Design review of the part built by this model. Coordinates are the model's own, in mm. Coordinates: 2 decimals unless noted, no trailing zeros. Loops run counter-clockwise (first coordinate to the right, second up) from the corner with the lowest first, then second, coordinate; pieces in that order, holes last. Notation, with made-up numbers: (59.25, -6) -> (99.25, -6) arc R28 ccw to (99.25, 15) -> close; hole circle Ø7 at (-8.5, 31.5). An arc over 180 degrees is marked (long way). Use one line per item in the form item = value. Start each with the question number.
1. Consider section B-B (y = 0.85). State the section outline as (x, z) points.
2. Wall thickness on line 1 (X direction, y = 0.45, z = -3); line 2 (Z direction, x = 19.5, y = 0.25); line 3 (X direction, y = 0.25, z = -29): over which ranges is each line inside the solid? List them lowest first. Write a range as from..to.
3. Consider section C-C (z = -3). State the section outline as (x, y) points.
4. Consider section A-A (x = 35.5). State the section outline as (y, z) points, then the cut area to 3 significant figures.
5. The part is to be moulded in two halves that separate along X. For faces 1 (the face through (24.2, 0, -23.8)), 2 (the face through (3.24, 0.49, -43.01)), 3 (the face through (46.24, 0.49, -43.84)), say which applies: released by +X, released by -X, zero draft, split by the parting line, or undercut.
from build123d import *

# Parameters (mm, degrees)
CROQUIS1_W                                 = 49
CROQUIS1_H                                 = 47
SALIENTE_EXTRUIR1_DEPTH                    = 1
PERFORADOR_PARA_ROSCAR_PARA_MACHO_DE_ROS_D = 2.5
CORTAR_EXTRUIR1_REACH                      = 69.904
CROQUIS5_W                                 = 30
CROQUIS5_H                                 = 8


with BuildPart() as part:
    # Croquis1 → Saliente-Extruir1 (new body)
    with BuildSketch(Plane(origin=(0, 0, 0), x_dir=(1, 0, 0), z_dir=(0, 1, 0))):
        with Locations((24.5, 23.5)):
            Rectangle(CROQUIS1_W, CROQUIS1_H)
    extrude(amount=SALIENTE_EXTRUIR1_DEPTH)

    # Perforador para roscar para macho de roscar para M31 (through all)
    with Locations(Plane(origin=(4, 1, -44), x_dir=(0, 0, 1), z_dir=(0, 1, 0))):
        with Locations((0, 0), (41, 0), (41, 41), (0, 41)):
            Hole(PERFORADOR_PARA_ROSCAR_PARA_MACHO_DE_ROS_D / 2)

    # Croquis5 → Cortar-Extruir1 (cut, up to next)
    with BuildSketch(Plane(origin=(0, 1, 0), x_dir=(1, 0, 0), z_dir=(0, 1, 0)), mode=Mode.PRIVATE) as cortar_extruir1_sk1:
        with Locations((24.5, 17)):
            Rectangle(CROQUIS5_W, CROQUIS5_H)
    cortar_extruir1_tool1 = extrude(cortar_extruir1_sk1.sketch, amount=-CORTAR_EXTRUIR1_REACH, mode=Mode.PRIVATE) & part.part
    # Croquis5 → Cortar-Extruir1 (cut, up to next)
    with BuildSketch(Plane(origin=(0, 1, 0), x_dir=(1, 0, 0), z_dir=(0, 1, 0)), mode=Mode.PRIVATE) as cortar_extruir1_sk2:
        with Locations((24.5, 28)):
            Rectangle(CROQUIS5_W, CROQUIS5_H)
    cortar_extruir1_tool2 = extrude(cortar_extruir1_sk2.sketch, amount=-CORTAR_EXTRUIR1_REACH, mode=Mode.PRIVATE) & part.part
    add(cortar_extruir1_tool1.solids().sort_by_distance((24.5, 1, -17))[0], mode=Mode.SUBTRACT)
    add(cortar_extruir1_tool2.solids().sort_by_distance((24.5, 1, -28))[0], mode=Mode.SUBTRACT)


solid = part.part
Geometry check:
q1.outline = (0, -47) -> (49, -47) -> (49, 0) -> (0, 0) -> close; hole circle Ø2.5 at (4, -44); hole circle Ø2.5 at (4, -3); hole (9.5, -32) -> (39.5, -32) -> (39.5, -24) -> (9.5, -24) -> close; hole (9.5, -21) -> (39.5, -21) -> (39.5, -13) -> (9.5, -13) -> close; hole circle Ø2.5 at (45, -44); hole circle Ø2.5 at (45, -3)
q2.line_1 = 0..2.75, 5.25..43.75, 46.25..49
q2.line_2 = -47..-32, -24..-21, -13..0
q2.line_3 = 0..9.5, 39.5..49
q3.outline = (0, 0) -> (2.75, 0) -> (2.75, 1) -> (0, 1) -> close; (5.25, 0) -> (43.75, 0) -> (43.75, 1) -> (5.25, 1) -> close; (46.25, 0) -> (49, 0) -> (49, 1) -> (46.25, 1) -> close
q4.outline = (0, -47) -> (1, -47) -> (1, -32) -> (0, -32) -> close; (0, -24) -> (1, -24) -> (1, -21) -> (0, -21) -> close; (0, -13) -> (1, -13) -> (1, 0) -> (0, 0) -> close
q4.area = 31.0 mm²
q5.face_1 = zero draft
q5.face_2 = undercut
q5.face_3 = undercut
